Here's how the part is built. I have some questions about the finished solid (model axes, mm). A direction names the side the tool comes from. Round coordinates to 2 decimals unless told otherwise and drop trailing zeros. Write each loop counter-clockwise with the first axis right and the second up, starting at its lowest first coordinate (ties: lowest second). Pieces come first, ordered by that corner, then holes. Notation, with made-up numbers: (88, 2) -> (99, 2) arc R19 cw to (99, 7) -> close; hole circle Ø10 at (81.5, -15). An arc over 180 degrees is marked (long way). Answer in a Markdown table with one row per item.
from build123d import *

# Parameters (mm, degrees)
SKETCH3_W            = 30
SKETCH3_H            = 30
BOSS_EXTRUDE1_DEPTH  = 40
CUT_EXTRUDE1_DEPTH   = 10
CUT_EXTRUDE2_DEPTH   = 5
CUT_EXTRUDE3_DEPTH   = 28
CUT_EXTRUDE4_START   = -40
CUT_EXTRUDE4_DEPTH   = 99.309519017
MIRROR5_START        = -40
MIRROR5_COPY_1_DEPTH = 99.309519017
SKETCH9_R            = 6
BOSS_EXTRUDE2_DEPTH  = 30
CUT_EXTRUDE5_DEPTH   = 30
SKETCH11_W           = 21.329134953
SKETCH11_H           = 5.145955698
CUT_EXTRUDE6_DEPTH   = 30


with BuildPart() as part:
    # Sketch3 → Boss-Extrude1 (new body)
    with BuildSketch(Plane.XY):
        with Locations((15, 15)):
            Rectangle(SKETCH3_W, SKETCH3_H)
    extrude(amount=BOSS_EXTRUDE1_DEPTH)

    # Sketch4 → Cut-Extrude1 (cut)
    with BuildSketch(Plane.XY.offset(40)):
        with BuildLine():
            ThreePointArc((20.75, 15), (17.200429736, 20.312307312), (10.934136008, 19.065863992))
            Line((10.934136008, 19.065863992), (19.065863992, 10.934136008))
            ThreePointArc((19.065863992, 10.934136008), (20.312307312, 12.799570264), (20.75, 15))
        make_face()
        with BuildLine():
            Line((19.065863992, 10.934136008), (10.934136008, 19.065863992))
            ThreePointArc((10.934136008, 19.065863992), (10.934136008, 10.934136008), (19.065863992, 10.934136008))
        make_face()
    extrude(amount=-CUT_EXTRUDE1_DEPTH, mode=Mode.SUBTRACT)

    # Sketch5 → Cut-Extrude2 (cut)
    with BuildSketch(Plane.XZ):
        Polygon((15, 38.58), (11.899629054, 36.79), (11.899629054, 33.21), (15, 31.42), (18.100370946, 33.21), (18.100370946, 36.79), align=None)
    cut_extrude2 = extrude(amount=-CUT_EXTRUDE2_DEPTH, mode=Mode.SUBTRACT)

    # Mirror1: Cut-Extrude2 across plane
    add(cut_extrude2.mirror(Plane(origin=(0, 15, 0), x_dir=(0, 0, 1), z_dir=(0, -1, 0))), mode=Mode.SUBTRACT)

    # Sketch6 → Cut-Extrude3 (cut)
    with BuildSketch(Plane(origin=(0, 25, 0), x_dir=(1, 0, 0), z_dir=(0, 1, 0))):
        with BuildLine():
            ThreePointArc((15, -33.25), (13.25, -35), (15, -36.75))
            Line((15, -36.75), (15, -33.25))
        make_face()
        with BuildLine():
            Line((15, -33.25), (15, -36.75))
            ThreePointArc((15, -36.75), (16.237436867, -36.237436867), (16.75, -35))
            ThreePointArc((16.75, -35), (16.237436867, -33.762563133), (15, -33.25))
        make_face()
    extrude(amount=-CUT_EXTRUDE3_DEPTH, mode=Mode.SUBTRACT)

    # Sketch8 → Cut-Extrude4 (cut)
    with BuildSketch(Plane(origin=(0, 0, 0), x_dir=(-1, 0, 0), z_dir=(0, 0, -1)).offset(CUT_EXTRUDE4_START)):
        Polygon((-77.236567429, -51.703622198), (-30, 17.572977849), (-21.526577959, 30), (25.70998947, 99.276600047), (-112.843210625, 193.749734905), (-215.789767524, 42.769512659), align=None)
    cut_extrude4 = extrude(amount=CUT_EXTRUDE4_DEPTH, mode=Mode.SUBTRACT)

    # Mirror4: Cut-Extrude4 across plane
    add(cut_extrude4.mirror(Plane.ZY.offset(-15)), mode=Mode.SUBTRACT)

    # Mirror5: Cut-Extrude4 across plane
    add(cut_extrude4.mirror(Plane(origin=(0, 15, 0), x_dir=(0, 0, 1), z_dir=(0, -1, 0))), mode=Mode.SUBTRACT)

    # Mirror5 copy 1 sketch → Mirror5 copy 1 (cut)
    with BuildSketch(Plane(origin=(30, 30, 0), x_dir=(1, 0, 0), z_dir=(0, 0, -1)).offset(MIRROR5_START)):
        Polygon((-77.236567429, -51.703622198), (-30, 17.572977849), (-21.526577959, 30), (25.70998947, 99.276600047), (-112.843210625, 193.749734905), (-215.789767524, 42.769512659), align=None)
    extrude(amount=MIRROR5_COPY_1_DEPTH, mode=Mode.SUBTRACT)

    # Sketch9 → Boss-Extrude2 (add)
    with BuildSketch(Plane(origin=(0, 0, 0), x_dir=(1, 0, 0), z_dir=(0, 1, 0))):
        with BuildLine():
            Line((5.769230769, 13.846153846), (0, 0))
            Line((0, 0), (30, 0))
            Line((30, 0), (24.424045098, 13.344753204))
            Line((24.424045098, 13.344753204), (24.002162862, 14.354430365))
            ThreePointArc((24.002162862, 14.354430365), (14.721339861, 19.996116672), (5.769230769, 13.846153846))
        make_face()
        with Locations(Location((15, 10, 0), (0, 0, 270))):
            Circle(SKETCH9_R, mode=Mode.SUBTRACT)
    extrude(amount=BOSS_EXTRUDE2_DEPTH)

    # Sketch10 → Cut-Extrude5 (cut)
    with BuildSketch(Plane.XY):
        Polygon((0, 17.572977849), (8.473422041, 30), (0, 30), align=None)
        Polygon((8.473422041, 0), (0, 0), (0, 12.427022151), align=None)
        Polygon((21.526577959, 0), (30, 12.427022151), (30, 0), align=None)
        Polygon((30, 17.572977849), (21.526577959, 30), (30, 30), align=None)
    extrude(amount=-CUT_EXTRUDE5_DEPTH, mode=Mode.SUBTRACT)

    # Sketch11 → Cut-Extrude6 (cut)
    with BuildSketch(Plane(origin=(30, 0, 0), x_dir=(0, 0, -1), z_dir=(1, 0, 0))):
        with Locations((10.664567477, 15)):
            Rectangle(SKETCH11_W, SKETCH11_H)
    extrude(amount=-CUT_EXTRUDE6_DEPTH, mode=Mode.SUBTRACT)


solid = part.part
1) I want a section at A-A, the plane y = 6.25. List the corners of the cut face in (x, z) for me, and give its area (3 significant figures).
Response:
| item | result |
|---|---|
| outline | (4.21, -10.11) -> (5.77, -13.85) arc R10 ccw to (24, -14.35) -> (25.79, -10.08) -> (25.79, 40) -> (4.21, 40) -> close; hole circle Ø12 at (15, -10); hole circle Ø3.5 at (15, 35) |
| area | 1,120 mm^2 |
2) I want a section at B-B, the plane z = 22.5. List the corners of the cut face in (x, y) for me.
Response:
| item | result |
|---|---|
| outline | (0, 12.43) -> (8.47, 0) -> (21.53, 0) -> (30, 12.43) -> (30, 17.57) -> (21.53, 30) -> (8.47, 30) -> (0, 17.57) -> close |
3) I need wall thicknesses on line 1 (Z direction, x = 15, y = 26.5); line 2 (X direction, y = 16.75, z = 31.5); line 3 (Z direction, x = 13, y = 2). Which ranges of each line are inside material? Lowest first, please. Write a range as [from, to].
Response:
| item | result |
|---|---|
| line 1 | z = [-20, -16], [-4, 31.42], [38.58, 40] |
| line 2 | x = [0, 9.52], [20.48, 30] |
| line 3 | z = [-19.8, -15.66], [-4.34, 32.57], [37.43, 40] |
4) I want a section at C-C, the plane z = -15. List the corners of the cut face in (x, y) for me, and give its area (3 significant figures).
Response:
| item | result |
|---|---|
| outline | (6.34, 3.13) -> (8.47, 0) -> (11.68, 0) -> (11.68, 12.43) -> (6.34, 12.43) -> close; (6.34, 17.57) -> (11.68, 17.57) -> (11.68, 30) -> (8.47, 30) -> (6.34, 26.87) -> close; (18.32, 0) -> (21.53, 0) -> (23.66, 3.13) -> (23.66, 12.43) -> (18.32, 12.43) -> close; (18.32, 17.57) -> (23.66, 17.57) -> (23.66, 26.87) -> (21.53, 30) -> (18.32, 30) -> close |
| area | 252 mm^2 |
5) We'd pull the mould along Y, two halves only. Please class faces 1 (the face through (15, 15, 0)), 2 (the face through (11.9, 28, 35)), 3 (the face through (15, 15, 30)), 4 (the face through (4.18, 6.3, 11.61)): +Y half, -Y half, draft (parallel to the pull), parting line (faces both ways), or undercut.
Response:
| item | result |
|---|---|
| face 1 | undercut |
| face 2 | draft |
| face 3 | undercut |
| face 4 | -Y half |
6) I want a section at D-D, the plane y = 23.5. List the corners of the cut face in (x, z) for me, and give its area (3 significant figures).
Response:
| item | result |
|---|---|
| outline | (4.04, -9.7) -> (5.77, -13.85) arc R10 ccw to (24, -14.35) -> (25.96, -9.67) -> (25.96, 40) -> (4.04, 40) -> close; hole circle Ø12 at (15, -10); hole circle Ø3.5 at (15, 35) |
| area | 1,130 mm^2 |
7) Which directions (+Z, -Z, +X, -X, +Y, -Y) give clear straight access to the entire face, cutting with the end or side of a thin tool? Please do faces 5 (the face through (11.9, 2, 35)), 6 (the face through (15, 30, 10)), 7 (the face through (16, 25, 37)).
Response:
| item | result |
|---|---|
| face 5 | -Y |
| face 6 | +Z, -Z, +X, -X, +Y |
| face 7 | +Y |
8) For pin 1 (1.1 mm diameter, centred on y = 27.5, z = 35.5, fed in from +X); pin 2 (2 mm diameter, centred on x = 9, y = 15.5, fed in from -Z); pin 3 (9.5 mm diameter, centred on x = 15, z = -10, fed in from +Y); pin 4 (3 mm diameter, centred on y = 3, z = 34.5, fed in from +X), each with a flat end and sliding along its axis, tell me the tip position at first contact or that it passes through.
Response:
| item | result |
|---|---|
| pin 1 | stops at x = 23.61 |
| pin 2 | stops at z = 0 |
| pin 3 | passes through |
| pin 4 | stops at x = 24.59 |
